Could you check a few things on this model? Use its own coordinates, in mm. Face numbers are marked on the shaded views. A direction names the side the tool comes from. Round coordinates to 2 decimals unless told otherwise and drop trailing zeros. Write each loop counter-clockwise with the first axis right and the second up, starting at its lowest first coordinate (ties: lowest second). Pieces come first, ordered by that corner, then holes. Notation, with made-up numbers: (-17, -30) -> (5, -30) arc R21 cw to (5, -1) -> close; hole circle Ø8 at (-22.5, 25.25). An arc over 180 degrees is marked (long way). One line per question, with ' | ' between items. Start each with the question number.
1. Imagine slicing it at A-A, the plane x = 8.5. List the corners of the cut face in (y, z) for me.
2. Imagine slicing it at C-C, the plane y = 1. State how many separate pieces and enclosed holes the cut face has, and give its area (3 significant figures).
3. Imagine slicing it at B-B, the plane z = -1.25. List the corners of the cut face in (x, y) for me.
4. For the marked faces 4, 5 and 6, which set-ups out of +Z, -Z, +X, -X, +Y, -Y let a thin tool reach every point of the face, with its end or its side?
5. Imagine slicing it at D-D, the plane z = 4.5. List the corners of the cut face in (x, y) for me, and give its area (3 significant figures).
6. If I drill on line 1 along Y through (x, z) = (-8.5, 1); line 2 along X through (y, z) = (0.75, -1.25); line 3 along X through (y, z) = (-4, 6.5), over which ranges is the centre line in solid material (lowest first)? Write a range as [from, to].
7. Thinking about a two-plate mould opening in X: for the marked faces 1, 2 and 3, which applies, released by +X, released by -X, zero draft, split by the parting line, or undercut?
8. For pin 1 Ø4.5 at (x, y) = (8.5, 0) entering from +Z; pin 2 Ø2 at (x, y) = (-5.5, -5.5) entering from +Z; pin 3 Ø3 at (y, z) = (-2.5, 4.5) entering from -X, each with a flat end and sliding along its axis, tell me the tip position at first contact or that it passes through.
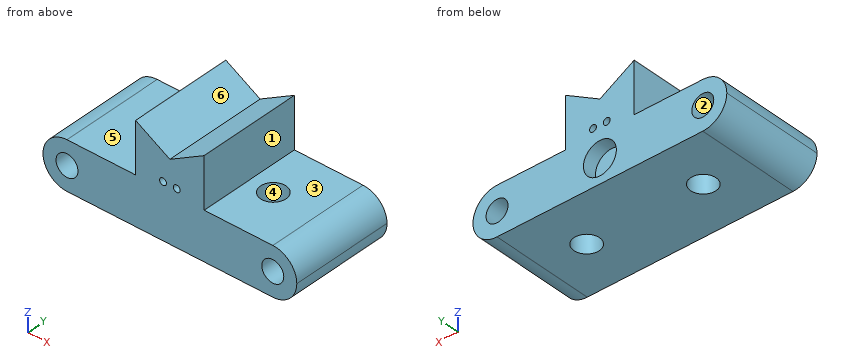
from build123d import *

# Parameters (mm, degrees)
SKIZZE1_W                       = 37
SKIZZE1_H                       = 7
SKIZZE1_R                       = 2.4
SKIZZE1_R_2                     = 1.6
SKIZZE1_R_3                     = 0.5
AUFSATZ_LINEAR_AUSTRAGEN1_DEPTH = 7.5
VERRUNDUNG1_R                   = 3.5
SKIZZE2_R                       = 1.85
SCHNITT_LINEAR_AUSTRAGEN1_DEPTH = 25.606475048
SKIZZE3_R                       = 2.4
SCHNITT_LINEAR_AUSTRAGEN2_DEPTH = 2


with BuildPart() as part:
    # Skizze1 → Aufsatz-Linear austragen1 (new, symmetric)
    # profile 1 of 3: a face of its own
    with BuildSketch(Plane(origin=(0, 0, 0), x_dir=(1, 0, 0), z_dir=(0, 1, 0))):
        Rectangle(SKIZZE1_W, SKIZZE1_H)
        Circle(SKIZZE1_R, mode=Mode.SUBTRACT)
        with Locations(Location((15, 0, 0), (0, 0, 270))):
            Circle(SKIZZE1_R_2, mode=Mode.SUBTRACT)
        with Locations(Location((-15, 0, 0), (0, 0, 270))):
            Circle(SKIZZE1_R_2, mode=Mode.SUBTRACT)
    # profile 2 of 3: a face of its own
    with BuildSketch(Plane(origin=(0, 0, 0), x_dir=(1, 0, 0), z_dir=(0, 1, 0))):
        Circle(SKIZZE1_R)
    # profile 3 of 3: a face of its own
    with BuildSketch(Plane(origin=(0, 0, 0), x_dir=(1, 0, 0), z_dir=(0, 1, 0))):
        Polygon((5, -3.5), (-5, -3.5), (-5, -10.886751346), (0, -8), (5, -10.886751346), align=None)
        with Locations(Location((-1, -4.5, 0), (0, 0, 270))):
            Circle(SKIZZE1_R_3, mode=Mode.SUBTRACT)
        with Locations(Location((1, -4.5, 0), (0, 0, 270))):
            Circle(SKIZZE1_R_3, mode=Mode.SUBTRACT)
    extrude(amount=AUFSATZ_LINEAR_AUSTRAGEN1_DEPTH, both=True)

    # Verrundung1
    verrundung1_edges = [part.edges().sort_by_distance(p)[0] for p in [
        (-18.5, 0, 3.5),
        (-18.5, 0, -3.5),
        (18.5, 0, -3.5),
        (18.5, 0, 3.5),
    ]]
    fillet(verrundung1_edges, radius=VERRUNDUNG1_R - 0.0001)  # a hair under: the kernel refuses the full size

    # Skizze2 → Schnitt-Linear austragen1 (cut, through all)
    with BuildSketch(Plane(origin=(0, 0, -3.5), x_dir=(-1, 0, 0), z_dir=(0, 0, -1))):
        with Locations((-8.5, 0)):
            Circle(SKIZZE2_R)
        with Locations((8.5, 0)):
            Circle(SKIZZE2_R)
    extrude(amount=-SCHNITT_LINEAR_AUSTRAGEN1_DEPTH, mode=Mode.SUBTRACT)

    # Skizze3 → Schnitt-Linear austragen2 (cut)
    with BuildSketch(Plane(origin=(0, 7.5, 0), x_dir=(1, 0, 0), z_dir=(0, 1, 0))):
        with Locations(Location((0, 0, 0), (0, 0, 270))):
            Circle(SKIZZE3_R)
    extrude(amount=-SCHNITT_LINEAR_AUSTRAGEN2_DEPTH, mode=Mode.SUBTRACT)


solid = part.part
Geometry results:
1) outline: (-7.5, -3.5) -> (-1.85, -3.5) -> (-1.85, 3.5) -> (-7.5, 3.5) -> close; (1.85, -3.5) -> (7.5, -3.5) -> (7.5, 3.5) -> (1.85, 3.5) -> close
2) separate pieces: 3 | enclosed holes: 4 | area: 247 mm2
3) outline: (-18.27, -7.5) -> (-16, -7.5) -> (-16, 7.5) -> (-18.27, 7.5) -> close; (-14, -7.5) -> (14, -7.5) -> (14, 7.5) -> (2.05, 7.5) -> (2.05, 5.5) -> (-2.05, 5.5) -> (-2.05, 7.5) -> (-14, 7.5) -> close; (16, -7.5) -> (18.27, -7.5) -> (18.27, 7.5) -> (16, 7.5) -> close; hole circle Ø3.7 at (-8.5, 0); hole circle Ø3.7 at (8.5, 0)
4) face 4: +Z, -Z | face 5: +Z, -X, +Y, -Y | face 6: +Z, +Y, -Y
5) outline: (-5, -7.5) -> (-1.5, -7.5) -> (-1.5, 7.5) -> (-5, 7.5) -> close; (-0.5, -7.5) -> (0.5, -7.5) -> (0.5, 7.5) -> (-0.5, 7.5) -> close; (1.5, -7.5) -> (5, -7.5) -> (5, 7.5) -> (1.5, 7.5) -> close | area: 120 mm2
6) line 1: y = [-7.5, -1.85], [1.85, 7.5] | line 2: x = [-18.27, -16], [-14, -10.19], [-6.81, 6.81], [10.19, 14], [16, 18.27] | line 3: x = [-5, 5]
7) face 1: released by +X | face 2: undercut | face 3: zero draft
8) pin 1: stops at z = 3.5 | pin 2: stops at z = 10.89 | pin 3: stops at x = -16.8
